The model under review builds one solid part; all positions refer to its coordinate system, in mm. Face numbers are marked on the shaded views. A direction names the side the tool comes from. Give positions to 0.01 mm unless a question says otherwise; leave off trailing zeros. Write each loop counter-clockwise with the first axis right and the second up, starting at its lowest first coordinate (ties: lowest second). Pieces come first, ordered by that corner, then holes. Notation, with made-up numbers: (-15, 21) -> (2, 21) arc R14 cw to (2, 42) -> close; hole circle Ø2 at (-39.75, 33.25). An arc over 180 degrees is marked (long way). Use CSV: the item, a comma, the result in double quotes.
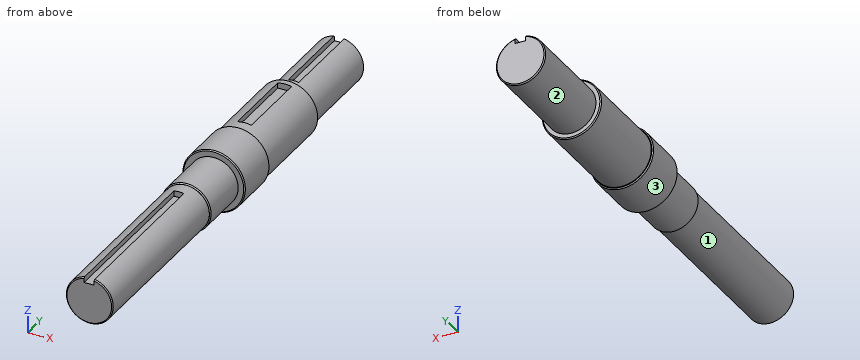
```python
from build123d import *

# Parameters (mm, degrees)
F0_W     = 168
F0_H     = 21.43
F0_W_2   = 44.5
F0_H_2   = 22.5
F0_W_3   = 44
F3_DEPTH = 156
F5_W     = 12.7
F5_H     = 7
F6_DEPTH = 70
F8_DEPTH = 80
F9_SIZE  = 1
F10_SIZE = 1
F11_SIZE = 1
F12_SIZE = 1


with BuildPart() as f1:
    # F0 (on Right) → F1 (revolve)
    with BuildSketch(Plane.YZ):
        with Locations((-132, 10.715)):
            Rectangle(F0_W, F0_H)
        Polygon((-48, 21.43), (-48, 0), (0, 0), (0, 22.5), (-48, 22.5), align=None)
        Polygon((0, 22.5), (0, 0), (43, 0), (43, 27.05), (43, 28.6), (0, 28.6), align=None)
        Polygon((43, 27.05), (43, 0), (130.5, 0), (130.5, 22.5), (130.5, 27.05), align=None)
        with Locations((152.75, 11.25)):
            Rectangle(F0_W_2, F0_H_2)
        with Locations((197, 11.25)):
            Rectangle(F0_W_3, F0_H_2)
    revolve(axis=Axis((0, 197, 0), (0, 1, 0)))

    # F2 (on face) → F3 (cut)
    with BuildSketch(Plane.XZ.offset(216)):
        with BuildLine():
            Line((-4.7436739586, 16), (4.4563260414, 16))
            Line((4.4563260414, 16), (4.4563260414, 20.9615375918))
            ThreePointArc((4.4563260414, 20.9615375918), (-0.1471030174, 21.4294951108), (-4.7436739586, 20.8983840852))
            Line((-4.7436739586, 20.8983840852), (-4.7436739586, 16))
        make_face()
    extrude(amount=-F3_DEPTH, mode=Mode.SUBTRACT)

    # F5 (on offset) → F6 (cut)
    with BuildSketch(Plane.XZ.offset(-54)):
        with Locations((-0.2053595381, 24.9309174805)):
            Rectangle(F5_W, F5_H)
    extrude(amount=-F6_DEPTH, mode=Mode.SUBTRACT)

    # F7 (on face) → F8 (cut)
    with BuildSketch(Plane(origin=(0, 219, 0), x_dir=(-1, 0, 0), z_dir=(0, 1, 0))):
        with BuildLine():
            ThreePointArc((4.76, 21.9907344125), (0, 22.5), (-4.76, 21.9907344125))
            Line((-4.76, 21.9907344125), (-4.76, 17.0498597833))
            Line((-4.76, 17.0498597833), (4.76, 17.0498597833))
            Line((4.76, 17.0498597833), (4.76, 21.9907344125))
        make_face()
    extrude(amount=-F8_DEPTH, mode=Mode.SUBTRACT)

    # F9
    f9_edges = [f1.edges().sort_by_distance(p)[0] for p in [
        (0.147103, -216, -21.429495),
    ]]
    chamfer(f9_edges, length=F9_SIZE)

    # F10
    f10_edges = [f1.edges().sort_by_distance(p)[0] for p in [
        (0, -48, -22.5),
    ]]
    chamfer(f10_edges, length=F10_SIZE)

    # F11
    f11_edges = [f1.edges().sort_by_distance(p)[0] for p in [
        (0, 0, -28.6),
        (0, 43, -28.6),
    ]]
    chamfer(f11_edges, length=F11_SIZE)

    # F12
    f12_edges = [f1.edges().sort_by_distance(p)[0] for p in [
        (0, 130.5, -27.05),
        (0, 219, -22.5),
    ]]
    chamfer(f12_edges, length=F12_SIZE)


solid = f1.part
```
Q1. To check wall thickness, follow probe 1 along Y at (x, z) = (-5, -22); probe 2 along X at (y, z) = (101, 1.5); probe 3 along X at (y, z) = (7.5, 20). State the ranges of each line that lie inside material, in increasing order.
Derived:
probe 1,"y = 0 to 130.5"
probe 2,"x = -27.01 to 27.01"
probe 3,"x = -20.44 to 20.44"
Q2. Consider section C-C (y = -131.5). Write out the cut boundary in (x, z), then the cut area to 3 significant figures.
Derived:
outline,"(-4.74, 16) -> (-4.74, 20.9) arc R21.43 ccw (long way) to (4.46, 20.96) -> (4.46, 16) -> close"
area,"1,390 mm2"
Q3. Insertion check: pin 1 (4 mm diameter, centred on x = -1.5, y = 87, fed in from +Z); pin 2 (10 mm diameter, centred on x = 1, y = -140.5, fed in from +Z); pin 3 (1.5 mm diameter, centred on y = -138.5, z = 19.5, fed in from +X). Each pin has a flat end and moves straight along its axis. Give the tip position at first contact, or say it passes through.
Derived:
pin 1,"stops at z = 21.43"
pin 2,"stops at z = 20.96"
pin 3,"stops at x = 10.38"
Q4. Consider section B-B (y = 7). Write out the cut boundary in (x, z).
Derived:
outline,"circle Ø57.2 at (0, 0)"
Q5. Machinability: for the marked faces 1, 2 and 3, which of the approach directions +Z, -Z, +X, -X, +Y, -Y give a long, thin tool a straight path to every point of the face, cutting with its end or side? Answer none if there is none.
Derived:
face 1,"-Y"
face 2,"+Y"
face 3,"+Y, -Y"
